The model under review builds one solid part; all positions refer to its coordinate system, in mm. A direction names the side the tool comes from. Round coordinates to 2 decimals unless told otherwise and drop trailing zeros. Loops run counter-clockwise (first coordinate to the right, second up) from the corner with the lowest first, then second, coordinate; pieces in that order, holes last. Notation, with made-up numbers: (-13, 41) - (-5, 41) arc R7 cw to (-5, 47) - close; hole circle Ø3 at (24.5, -32.5). An arc over 180 degrees is marked (long way). Answer as CSV lines item,"result".
from build123d import *

# Parameters (mm, degrees)
SKETCH1_W               = 300
SKETCH1_H               = 100
SKETCH1_R               = 2.5
BOSS_EXTRUDE1_DEPTH     = 10
SKETCH2_W               = 10
SKETCH2_H               = 50
BOSS_EXTRUDE2_DEPTH     = 260
SKETCH3_R               = 5.25
CUT_EXTRUDE1_DEPTH      = 20
CUT_EXTRUDE2_DEPTH      = 411.984872046
CUT_EXTRUDE2_DEPTH_BACK = 411.984872046
SKETCH5_R               = 1.5
CUT_EXTRUDE3_DEPTH      = 10
SKETCH7_R               = 1.5
CUT_EXTRUDE6_DEPTH      = 10
SKETCH8_R               = 1.5
CUT_EXTRUDE7_DEPTH      = 10
SKETCH12_R              = 6.25
BOSS_EXTRUDE4_DEPTH     = 27
CUT_EXTRUDE10_START     = -34
SKETCH13_R              = 5.25
CUT_EXTRUDE10_DEPTH     = 34


with BuildPart() as part:
    # Sketch1 → Boss-Extrude1 (new body)
    with BuildSketch(Plane(origin=(0, 0, 0), x_dir=(1, 0, 0), z_dir=(0, 1, 0))):
        with Locations((37.664745703, -59.126371929)):
            Rectangle(SKETCH1_W, SKETCH1_H)
        with Locations(Location((-97.335254297, -24.126371929, 0), (0, 0, 270))):
            Circle(SKETCH1_R, mode=Mode.SUBTRACT)
        with Locations(Location((-97.335254297, -94.126371929, 0), (0, 0, 90))):
            Circle(SKETCH1_R, mode=Mode.SUBTRACT)
        with Locations(Location((172.664745703, -24.126371929, 0), (0, 0, 90))):
            Circle(SKETCH1_R, mode=Mode.SUBTRACT)
        with Locations(Location((172.664745703, -94.126371929, 0), (0, 0, 270))):
            Circle(SKETCH1_R, mode=Mode.SUBTRACT)
    extrude(amount=BOSS_EXTRUDE1_DEPTH)

    # Sketch2 → Boss-Extrude2 (add)
    with BuildSketch(Plane(origin=(0, 10, 0), x_dir=(1, 0, 0), z_dir=(0, 1, 0))):
        with Locations((172.664745703, -58.546819536)):
            Rectangle(SKETCH2_W, SKETCH2_H)
        with Locations((-97.335254297, -58.546819536)):
            Rectangle(SKETCH2_W, SKETCH2_H)
    extrude(amount=BOSS_EXTRUDE2_DEPTH)

    # Sketch3 → Cut-Extrude1 (cut)
    with BuildSketch(Plane.ZY.offset(82.335254297)):
        with Locations((59.126371929, 250)):
            Circle(SKETCH3_R)
    extrude(amount=CUT_EXTRUDE1_DEPTH, mode=Mode.SUBTRACT)

    # Sketch4 → Cut-Extrude2 (cut, two sides: drawn at the far end of the back side and taken through both)
    with BuildSketch(Plane.ZY.offset(102.335254297).offset(-CUT_EXTRUDE2_DEPTH_BACK)):
        with BuildLine():
            Line((83.546819536, 270), (58.546819536, 270))
            ThreePointArc((58.546819536, 270), (74.165001003, 264.798991748), (83.546819536, 251.27273727))
            Line((83.546819536, 251.27273727), (83.546819536, 270))
        make_face()
        with BuildLine():
            Line((33.546819536, 270), (33.546819536, 251.27273727))
            ThreePointArc((33.546819536, 251.27273727), (42.928638069, 264.798991748), (58.546819536, 270))
            Line((58.546819536, 270), (33.546819536, 270))
        make_face()
    extrude(amount=CUT_EXTRUDE2_DEPTH + CUT_EXTRUDE2_DEPTH_BACK, mode=Mode.SUBTRACT)

    # Sketch5 → Cut-Extrude3 (cut)
    with BuildSketch(Plane.ZY.offset(102.335254297)):
        with Locations((58.546819536, 172.564056087)):
            Circle(SKETCH5_R)
        with Locations((58.546819536, 38.564056087)):
            Circle(SKETCH5_R)
    extrude(amount=-CUT_EXTRUDE3_DEPTH, mode=Mode.SUBTRACT)

    # Sketch7 → Cut-Extrude6 (cut)
    with BuildSketch(Plane.ZY.offset(102.335254297)):
        with Locations((59.126371929, 260)):
            Circle(SKETCH7_R)
        with Locations((59.126371929, 240)):
            Circle(SKETCH7_R)
    extrude(amount=-CUT_EXTRUDE6_DEPTH, mode=Mode.SUBTRACT)

    # Sketch8 → Cut-Extrude7 (cut)
    with BuildSketch(Plane.ZY.offset(102.335254297)):
        with Locations((50.626371929, 250)):
            Circle(SKETCH8_R)
        with Locations((67.626371929, 250)):
            Circle(SKETCH8_R)
    extrude(amount=-CUT_EXTRUDE7_DEPTH, mode=Mode.SUBTRACT)

    # Sketch12 → Boss-Extrude4 (add)
    with BuildSketch(Plane(origin=(177.664745703, 0, 0), x_dir=(0, 0, -1), z_dir=(1, 0, 0))):
        with Locations(Location((-59.126371929, 250, 0), (0, 0, 180))):
            Circle(SKETCH12_R)
    extrude(amount=BOSS_EXTRUDE4_DEPTH)

    # Sketch13 → Cut-Extrude10 (cut)
    with BuildSketch(Plane.ZY.offset(-167.664745703).offset(CUT_EXTRUDE10_START)):
        with Locations((59.126371929, 250)):
            Circle(SKETCH13_R)
    extrude(amount=CUT_EXTRUDE10_DEPTH, mode=Mode.SUBTRACT)


solid = part.part
1. Wall thickness on probe 1 along X at (y, z) = (211.5, 38); probe 2 along Z at (x, y) = (-96, 240); probe 3 along Y at (x, z) = (51.5, 40.5): over which ranges is each line inside the solid? List them lowest first.
Numbers:
probe 1,"x = -102.34 to -92.34, 167.66 to 177.66"
probe 2,"z = 33.55 to 57.63, 60.63 to 83.55"
probe 3,"y = 0 to 10"
2. Tool access review of faces 1 (the face through (190.976, 255.545, 62.01)), 2 (the face through (-102.335, 138, 59)), 3 (the face through (-97, 129, 83.547)), 4 (the face through (167.665, 138, 59)), 5 (the face through (201.665, 250, 59)): name each direction out of +Z, -Z, +X, -X, +Y, -Y from which nothing blocks a thin tool from reaching the whole face with its end or side.
Numbers:
face 1,"+X"
face 2,"+Z, -Z, -X, +Y"
face 3,"+Z, +X, -X, +Y"
face 4,"+Z, -Z, +Y"
face 5,"-X"
3. Draft analysis for pull direction Z (two halves, no side actions). For faces 6 (the face through (173, 129, 33.547)), 7 (the face through (-92.335, 138, 59)), 8 (the face through (36, 5, 109.126)), 9 (the face through (-97.27, 253.55, 55.26)), state which applies: +Z half, -Z half, draft (parallel to the pull), parting line (faces both ways), or undercut.
Numbers:
face 6,"-Z half"
face 7,"draft"
face 8,"+Z half"
face 9,"undercut"
4. Take a section at B-B (z = 15). State the section outline as (x, y) points.
Numbers:
outline,"(-112.34, 0) - (187.66, 0) - (187.66, 10) - (-112.34, 10) - close"
5. Take a section at A-A (y = 55). State the section outline as (x, z) points.
Numbers:
outline,"(-102.34, 33.55) - (-92.34, 33.55) - (-92.34, 83.55) - (-102.34, 83.55) - close; (167.66, 33.55) - (177.66, 33.55) - (177.66, 83.55) - (167.66, 83.55) - close"
6. Clearance check with flat-ended pins moving along their axes: pin 1 (2 mm diameter, centred on y = 161, z = 65, fed in from +X); pin 2 (12 mm diameter, centred on y = 176.5, z = 85, fed in from -X); pin 3 (12 mm diameter, centred on x = -2.5, z = 36.5, fed in from +Y). State where each tip first meets the part, or that it passes through.
Numbers:
pin 1,"stops at x = 177.66"
pin 2,"stops at x = -102.34"
pin 3,"stops at y = 10"
7. Take a section at C-C (x = 82.5). State the section outline as (y, z) points.
Numbers:
outline,"(0, 9.13) - (10, 9.13) - (10, 109.13) - (0, 109.13) - close"
